Input: part model. Units: mm. Frame: model coordinates. Coordinates: 2 decimals unless noted, no trailing zeros. Order: outer loops, then holes, each group sorted by start corner. A loop starts at its lowest first (then second) coordinate and runs counter-clockwise, first axis right, second up. Notation, with made-up numbers: (4.5, 76) - (17.5, 76) arc R23 cw to (17.5, 100) - close; hole circle Ø11 at (82, 58.5). An arc over 180 degrees is marked (long way). Use a Markdown table: item, result. Add a question column.
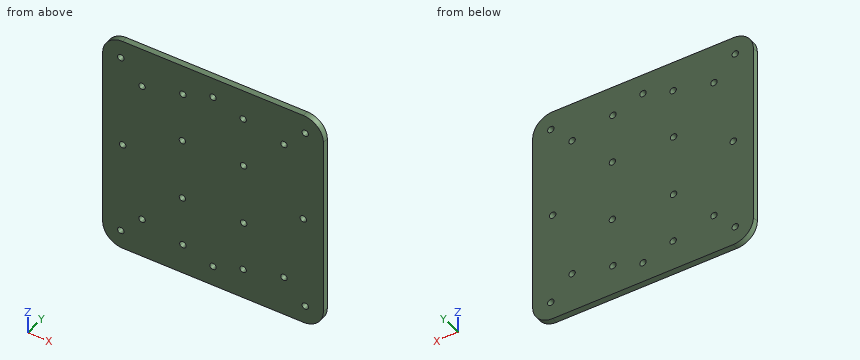
from build123d import *

# Parameters (mm, degrees)
SKETCH2_W           = 110
SKETCH2_H           = 110
SKETCH2_R           = 1.6
BOSS_EXTRUDE1_DEPTH = 3
FILLET1_R           = 10


with BuildPart() as part:
    # Sketch2 → Boss-Extrude1 (new body)
    with BuildSketch(Plane(origin=(0, 0, 0), x_dir=(1, 0, 0), z_dir=(0, 1, 0))):
        Rectangle(SKETCH2_W, SKETCH2_H)
        with Locations(Location((15.25, 15.25, 0), (0, 0, 270))):
            Circle(SKETCH2_R, mode=Mode.SUBTRACT)
        with Locations(Location((-15.25, 15.25, 0), (0, 0, 90))):
            Circle(SKETCH2_R, mode=Mode.SUBTRACT)
        with Locations(Location((-15.25, -15.25, 0), (0, 0, 270))):
            Circle(SKETCH2_R, mode=Mode.SUBTRACT)
        with Locations(Location((15.25, -15.25, 0), (0, 0, 90))):
            Circle(SKETCH2_R, mode=Mode.SUBTRACT)
        with Locations(Location((35.3553, 35.3553, 0), (0, 0, 270))):
            Circle(SKETCH2_R, mode=Mode.SUBTRACT)
        with Locations(Location((45.9619, 45.9619, 0), (0, 0, 270))):
            Circle(SKETCH2_R, mode=Mode.SUBTRACT)
        with Locations(Location((-35.3553, 35.3553, 0), (0, 0, 90))):
            Circle(SKETCH2_R, mode=Mode.SUBTRACT)
        with Locations(Location((-45.9619, 45.9619, 0), (0, 0, 90))):
            Circle(SKETCH2_R, mode=Mode.SUBTRACT)
        with Locations(Location((45.9619, -45.9619, 0), (0, 0, 90))):
            Circle(SKETCH2_R, mode=Mode.SUBTRACT)
        with Locations(Location((35.3553, -35.3553, 0), (0, 0, 90))):
            Circle(SKETCH2_R, mode=Mode.SUBTRACT)
        with Locations(Location((-45.9619, -45.9619, 0), (0, 0, 270))):
            Circle(SKETCH2_R, mode=Mode.SUBTRACT)
        with Locations(Location((-35.3553, -35.3553, 0), (0, 0, 270))):
            Circle(SKETCH2_R, mode=Mode.SUBTRACT)
        with Locations(Location((0, 45, 0), (0, 0, 270))):
            Circle(SKETCH2_R, mode=Mode.SUBTRACT)
        with Locations(Location((-45, 0, 0), (0, 0, 270))):
            Circle(SKETCH2_R, mode=Mode.SUBTRACT)
        with Locations(Location((45, 0, 0), (0, 0, 270))):
            Circle(SKETCH2_R, mode=Mode.SUBTRACT)
        with Locations(Location((0, -45, 0), (0, 0, 270))):
            Circle(SKETCH2_R, mode=Mode.SUBTRACT)
        with Locations(Location((-15, -40, 0), (0, 0, 270))):
            Circle(SKETCH2_R, mode=Mode.SUBTRACT)
        with Locations(Location((15, -40, 0), (0, 0, 270))):
            Circle(SKETCH2_R, mode=Mode.SUBTRACT)
        with Locations(Location((-15, 40, 0), (0, 0, 270))):
            Circle(SKETCH2_R, mode=Mode.SUBTRACT)
        with Locations(Location((15, 40, 0), (0, 0, 270))):
            Circle(SKETCH2_R, mode=Mode.SUBTRACT)
    extrude(amount=BOSS_EXTRUDE1_DEPTH)

    # Fillet1
    fillet1_edges = [part.edges().sort_by_distance(p)[0] for p in [
        (55, 1.5, 55),
        (-55, 1.5, 55),
        (-55, 1.5, -55),
        (55, 1.5, -55),
    ]]
    fillet(fillet1_edges, radius=FILLET1_R)


solid = part.part
1) Material intervals for L1, parallel to X at y = 2.05, z = -15.25; L2, parallel to X at y = 0.8, z = 0; L3, parallel to X at y = 0.75, z = 45, sorted ascending.
2) Cut plane B-B (z = -15.25). Return the cut outline in (x, y).
3) Cut plane C-C (y = 1.2). State how many separate pieces and enclosed holes the cut face has, and give its area (3 significant figures).
4) Cut plane A-A (x = 0). Return the cut outline in (y, z).
Computed:
| question | item | result |
|---|---|---|
| 1 | L1 | x = -55 to -16.85, -13.65 to 13.65, 16.85 to 55 |
| 1 | L2 | x = -55 to -46.6, -43.4 to 43.4, 46.6 to 55 |
| 1 | L3 | x = -55 to -47.24, -44.68 to -1.6, 1.6 to 44.68, 47.24 to 55 |
| 2 | outline | (-55, 0) - (-16.85, 0) - (-16.85, 3) - (-55, 3) - close; (-13.65, 0) - (13.65, 0) - (13.65, 3) - (-13.65, 3) - close; (16.85, 0) - (55, 0) - (55, 3) - (16.85, 3) - close |
| 3 | separate pieces | 1 |
| 3 | enclosed holes | 20 |
| 3 | area | 11,900 mm2 |
| 4 | outline | (0, -55) - (3, -55) - (3, -46.6) - (0, -46.6) - close; (0, -43.4) - (3, -43.4) - (3, 43.4) - (0, 43.4) - close; (0, 46.6) - (3, 46.6) - (3, 55) - (0, 55) - close |
